```python
from build123d import *

# Parameters (mm, degrees)
SKETCH1_W            = 70
SKETCH1_H            = 70
BOSS_EXTRUDE1_DEPTH  = 15
FILLET1_R            = 15
M3_CLEARANCE_HOLE1_D = 3.4
SKETCH4_R            = 7.5
CUT_EXTRUDE1_DEPTH   = 16
SKETCH5_W            = 30
SKETCH5_H            = 30
CUT_EXTRUDE2_DEPTH   = 2.5
SKETCH6_W            = 45
SKETCH6_H            = 45
CUT_EXTRUDE3_DEPTH   = 10


with BuildPart() as part:
    # Sketch1 → Boss-Extrude1 (new body)
    with BuildSketch(Plane.XY):
        Rectangle(SKETCH1_W, SKETCH1_H)
    extrude(amount=BOSS_EXTRUDE1_DEPTH)

    # Fillet1
    fillet1_edges = [part.edges().sort_by_distance(p)[0] for p in [
        (-35, 35, 7.5),
        (35, 35, 7.5),
        (35, -35, 7.5),
        (-35, -35, 7.5),
    ]]
    fillet(fillet1_edges, radius=FILLET1_R)

    # M3 Clearance Hole1 (through all)
    with Locations(Plane.XY.offset(15)):
        with Locations((-26, -26), (26, -26), (26, 26), (-26, 26)):
            Hole(M3_CLEARANCE_HOLE1_D / 2)

    # Sketch4 → Cut-Extrude1 (cut, through all)
    with BuildSketch(Plane.XY.offset(15)):
        Circle(SKETCH4_R)
    extrude(amount=-CUT_EXTRUDE1_DEPTH, mode=Mode.SUBTRACT)

    # Sketch5 → Cut-Extrude2 (cut)
    with BuildSketch(Plane.XY.offset(15)):
        Rectangle(SKETCH5_W, SKETCH5_H)
    extrude(amount=-CUT_EXTRUDE2_DEPTH, mode=Mode.SUBTRACT)

    # Sketch6 → Cut-Extrude3 (cut)
    with BuildSketch(Plane(origin=(0, 0, 0), x_dir=(-1, 0, 0), z_dir=(0, 0, -1))):
        Rectangle(SKETCH6_W, SKETCH6_H)
    extrude(amount=-CUT_EXTRUDE3_DEPTH, mode=Mode.SUBTRACT)


solid = part.part
```
Part model, mm, in its own coordinate system. A direction names the side the tool comes from. Round coordinates to 2 decimals unless told otherwise and drop trailing zeros. Write each loop counter-clockwise with the first axis right and the second up, starting at its lowest first coordinate (ties: lowest second). Pieces come first, ordered by that corner, then holes.
Item 1: Probe L1, parallel to X at y = 13, z = 6.75; L2, parallel to X at y = 12, z = 12.75. List the from-to ranges inside material, lowest first.
Results:
L1: x = -35 to -22.5, 22.5 to 35
L2: x = -35 to -15, 15 to 35
Item 2: Cut at A-A, the plane y = 0. Give the cut face in (x, z).
Results:
outline: (-35, 0) - (-22.5, 0) - (-22.5, 10) - (-7.5, 10) - (-7.5, 12.5) - (-15, 12.5) - (-15, 15) - (-35, 15) - close; (7.5, 10) - (22.5, 10) - (22.5, 0) - (35, 0) - (35, 15) - (15, 15) - (15, 12.5) - (7.5, 12.5) - close
Item 3: Cut at C-C, the plane z = 5.75. Give the cut face in (x, y), plus the area to 3 significant figures.
Results:
outline: (-35, -20) arc R15 ccw to (-20, -35) - (20, -35) arc R15 ccw to (35, -20) - (35, 20) arc R15 ccw to (20, 35) - (-20, 35) arc R15 ccw to (-35, 20) - close; hole circle Ø3.4 at (-26, -26); hole circle Ø3.4 at (-26, 26); hole (-22.5, -22.5) - (22.5, -22.5) - (22.5, 22.5) - (-22.5, 22.5) - close; hole circle Ø3.4 at (26, -26); hole circle Ø3.4 at (26, 26)
area: 2,650 mm2
Item 4: Two-plate mould, pull along X, no slides. Class faces 4 (the flat face through (0, -35, 7)), 5 (the flat face through (-35, 0, 7)), 6 (the cylindrical face through (-26.914, -24.567, 7.395)): +X half, -X half, draft (parallel to the pull), parting line (faces both ways), or undercut.
Results:
face 4: draft
face 5: -X half
face 6: undercut
Item 5: Drop flat-ended pins along their axis: pin 1 Ø3 at (x, y) = (13, 18.5) entering from -Z; pin 2 Ø9 at (x, y) = (-1.5, -5.5) entering from +Z; pin 3 Ø13.5 at (x, y) = (0, 0) entering from +Z. Give the stop position or say it passes through.
Results:
pin 1: stops at z = 10
pin 2: stops at z = 12.5
pin 3: passes through
Item 6: Which spindle directions (+Z, -Z, +X, -X, +Y, -Y) get a long thin tool onto all of the face, cutting with end or side? Do faces 1 (the flat face through (0, 35, 7)), 2 (the flat face through (22.5, 0, 5)), 3 (the flat face through (15, 0, 14)). Say none if no direction does.
Results:
face 1: +Z, -Z, +X, -X, +Y
face 2: -Z
face 3: +Z
Item 7: Cut at D-D, the plane y = 13. Give the cut face in (x, z), plus the area to 3 significant figures.
Results:
outline: (-35, 0) - (-22.5, 0) - (-22.5, 10) - (22.5, 10) - (22.5, 0) - (35, 0) - (35, 15) - (15, 15) - (15, 12.5) - (-15, 12.5) - (-15, 15) - (-35, 15) - close
area: 525 mm2
